Here's how the part is built. I have some questions about the finished solid (model axes, mm). A direction names the side the tool comes from. Round coordinates to 2 decimals unless told otherwise and drop trailing zeros. Write each loop counter-clockwise with the first axis right and the second up, starting at its lowest first coordinate (ties: lowest second). Pieces come first, ordered by that corner, then holes. Notation, with made-up numbers: (-9.5, 84) - (14.5, 84) arc R18 cw to (14.5, 97) - close; hole circle Ø11 at (54, -32). An arc over 180 degrees is marked (long way). Return JSON: item names as keys, results as strings. Group by question number.
```python
from build123d import *

# Parameters (mm, degrees)
F1_DEPTH = 3.175


# Not quite as in the source:
# - a length typed as a fraction of an inch, garbled in the dataset ("3 / 203.2 mm" for 3/8 in), is restored


with BuildPart() as f1:
    # F0 (on Front) → F1 (new body)
    with BuildSketch(Plane.XZ):
        with BuildLine():
            ThreePointArc((-43.3524121445, 26.4803391454), (-44.3048599399, -24.8539611673), (0, -50.8))
            ThreePointArc((0, -50.8), (44.3048599399, -24.8539611673), (43.3524121445, 26.4803391454))
            Line((43.3524121445, 26.4803391454), (57.15, 50.8))
            Line((57.15, 50.8), (50.8, 50.8))
            Line((50.8, 50.8), (3.175, 50.8))
            Line((3.175, 50.8), (3.175, 50.700684167))
            ThreePointArc((3.175, 50.700684167), (1.5882764743, 50.7751649711), (0, 50.8))
            ThreePointArc((0, 50.8), (-1.5882764743, 50.7751649711), (-3.175, 50.700684167))
            Line((-3.175, 50.700684167), (-3.175, 50.8))
            Line((-3.175, 50.8), (-50.8, 50.8))
            Line((-50.8, 50.8), (-57.15, 50.8))
            Line((-57.15, 50.8), (-43.3524121445, 26.4803391454))
        make_face()
        with BuildLine():
            Line((-39.6867141727, 20.0191712658), (-3.175, -44.336462139))
            ThreePointArc((-3.175, -44.336462139), (-38.6612664458, -21.9341965162), (-39.6867141727, 20.0191712658))
        make_face(mode=Mode.SUBTRACT)
        with BuildLine():
            ThreePointArc((39.6867141727, 20.0191712658), (38.6612664458, -21.9341965162), (3.175, -44.336462139))
            Line((3.175, -44.336462139), (39.6867141727, 20.0191712658))
        make_face(mode=Mode.SUBTRACT)
        with BuildLine():
            ThreePointArc((-36.429171038, 25.4699430208), (-21.9341965162, 38.6612664458), (-3.175, 44.336462139))
            Line((-3.175, 44.336462139), (-3.175, -33.1439371814))
            Line((-3.175, -33.1439371814), (-36.429171038, 25.4699430208))
        make_face(mode=Mode.SUBTRACT)
        with BuildLine():
            Line((-47.1973723398, 44.45), (-24.5934442484, 44.45))
            ThreePointArc((-24.5934442484, 44.45), (-32.8665744068, 38.7353622258), (-39.8520903437, 31.5031886519))
            Line((-39.8520903437, 31.5031886519), (-47.1973723398, 44.45))
        make_face(mode=Mode.SUBTRACT)
        with BuildLine():
            Line((3.175, -33.1439371814), (3.175, 44.336462139))
            ThreePointArc((3.175, 44.336462139), (21.9341965162, 38.6612664458), (36.429171038, 25.4699430208))
            Line((36.429171038, 25.4699430208), (3.175, -33.1439371814))
        make_face(mode=Mode.SUBTRACT)
        with BuildLine():
            ThreePointArc((39.8520903437, 31.5031886519), (32.8665744068, 38.7353622258), (24.5934442484, 44.45))
            Line((24.5934442484, 44.45), (47.1973723398, 44.45))
            Line((47.1973723398, 44.45), (39.8520903437, 31.5031886519))
        make_face(mode=Mode.SUBTRACT)
    extrude(amount=F1_DEPTH)


solid = f1.part
```
1) Imagine slicing it at A-A (z = -26). Please give me the cut outline in (x, y) (3 decimals), plus the area to 3 significant figures.
2) Imagine slicing it at B-B (y = -0.6). Please give me the cut outline in (x, z) (3 decimals), plus the area to 3 significant figures.
3) Will these pins go through, and if not, where does the flat tip stop? pin 1 Ø1 at (y, z) = (-1.5, 23) entering from +X; pin 2 Ø1 at (y, z) = (-1.5, 17.5) entering from -X; pin 3 Ø2 at (x, z) = (41, 39) entering from -Y; pin 4 Ø1.5 at (y, z) = (-2.5, 2.5) entering from -X.
4) Imagine slicing it at D-D (z = -10). Please give me the cut outline in (x, y) (3 decimals).
5) Imagine slicing it at C-C (x = 34). Please give me the cut outline in (y, z) (3 decimals), plus the area to 3 significant figures.
6) If we mould it in two halves opening along Z, with no side actions, what happens to faces 4 (the flat face through (-30, -2, 50.8)), 5 (the flat face through (-19.57, -1.57, -4.25)), 6 (the flat face through (0, -3.175, 12))? For each: released by +Z, released by -Z, zero draft, split by the parting line, or undercut.
7) For faces 1 (the flat face through (50.155, -1.565, 38.47)), 2 (the flat face through (31, -2, 50.8)), 3 (the flat face through (-21.686, -1.565, -11.708)), which set-ups out of +Z, -Z, +X, -X, +Y, -Y let a thin tool reach every point of the face, with its end or its side?
8) I need wall thicknesses on line 1 along Z through (x, y) = (24, -1.85); line 2 along Z through (x, y) = (-3.5, -1.5); line 3 along X through (y, z) = (-1.5, 40) (3 decimals). Which ranges of each line are inside material? Lowest first, please.
Results found:
{
 "1": {"outline": "(-43.642, -3.175) - (-36.053, -3.175) - (-36.053, 0) - (-43.642, 0) - close; (-13.578, -3.175) - (-7.228, -3.175) - (-7.228, 0) - (-13.578, 0) - close; (-3.175, -3.175) - (3.175, -3.175) - (3.175, 0) - (-3.175, 0) - close; (7.228, -3.175) - (13.578, -3.175) - (13.578, 0) - (7.228, 0) - close; (36.053, -3.175) - (43.642, -3.175) - (43.642, 0) - (36.053, 0) - close", "area": "109 mm²"},
 "2": {"outline": "(-57.15, 50.8) - (-43.352, 26.48) arc R50.8 ccw (long way) to (43.352, 26.48) - (57.15, 50.8) - (3.175, 50.8) - (3.175, 50.701) arc R50.8 ccw to (-3.175, 50.701) - (-3.175, 50.8) - close; hole (-47.197, 44.45) - (-39.852, 31.503) arc R50.8 cw to (-24.593, 44.45) - close; hole (-39.687, 20.019) arc R44.45 ccw to (-3.175, -44.336) - close; hole (-36.429, 25.47) - (-3.175, -33.144) - (-3.175, 44.336) arc R44.45 ccw to start; hole (3.175, -44.336) arc R44.45 ccw to (39.687, 20.019) - close; hole (3.175, -33.144) - (36.429, 25.47) arc R44.45 ccw to (3.175, 44.336) - close; hole (24.593, 44.45) arc R50.8 cw to (39.852, 31.503) - (47.197, 44.45) - close", "area": "3,930 mm²"},
 "3": {"pin 1": "stops at x = 45.55", "pin 2": "stops at x = -47.87", "pin 3": "passes through", "pin 4": "stops at x = -50.77"},
 "4": {"outline": "(-49.806, -3.175) - (-43.311, -3.175) - (-43.311, 0) - (-49.806, 0) - close; (-22.656, -3.175) - (-16.306, -3.175) - (-16.306, 0) - (-22.656, 0) - close; (-3.175, -3.175) - (3.175, -3.175) - (3.175, 0) - (-3.175, 0) - close; (16.306, -3.175) - (22.656, -3.175) - (22.656, 0) - (16.306, 0) - close; (43.311, -3.175) - (49.806, -3.175) - (49.806, 0) - (43.311, 0) - close"},
 "5": {"outline": "(-3.175, -37.744) - (0, -37.744) - (0, -28.632) - (-3.175, -28.632) - close; (-3.175, 9.996) - (0, 9.996) - (0, 21.188) - (-3.175, 21.188) - close; (-3.175, 28.632) - (0, 28.632) - (0, 37.744) - (-3.175, 37.744) - close; (-3.175, 44.45) - (0, 44.45) - (0, 50.8) - (-3.175, 50.8) - close", "area": "114 mm²"},
 "6": {"face 4": "released by +Z", "face 5": "undercut", "face 6": "zero draft"},
 "7": {"face 1": "+X, +Y, -Y", "face 2": "+Z, +X, -X, +Y, -Y", "face 3": "+Y, -Y"},
 "8": {"line 1": "z = -44.77 to -37.41, -7.63 to 3.56, 37.41 to 50.8", "line 2": "z = -50.68 to -44.31, -43.76 to -32.57, 44.31 to 50.8", "line 3": "x = -51.023 to -44.673, -31.315 to -19.386, -3.175 to 3.175, 19.386 to 31.315, 44.673 to 51.023"}
}
